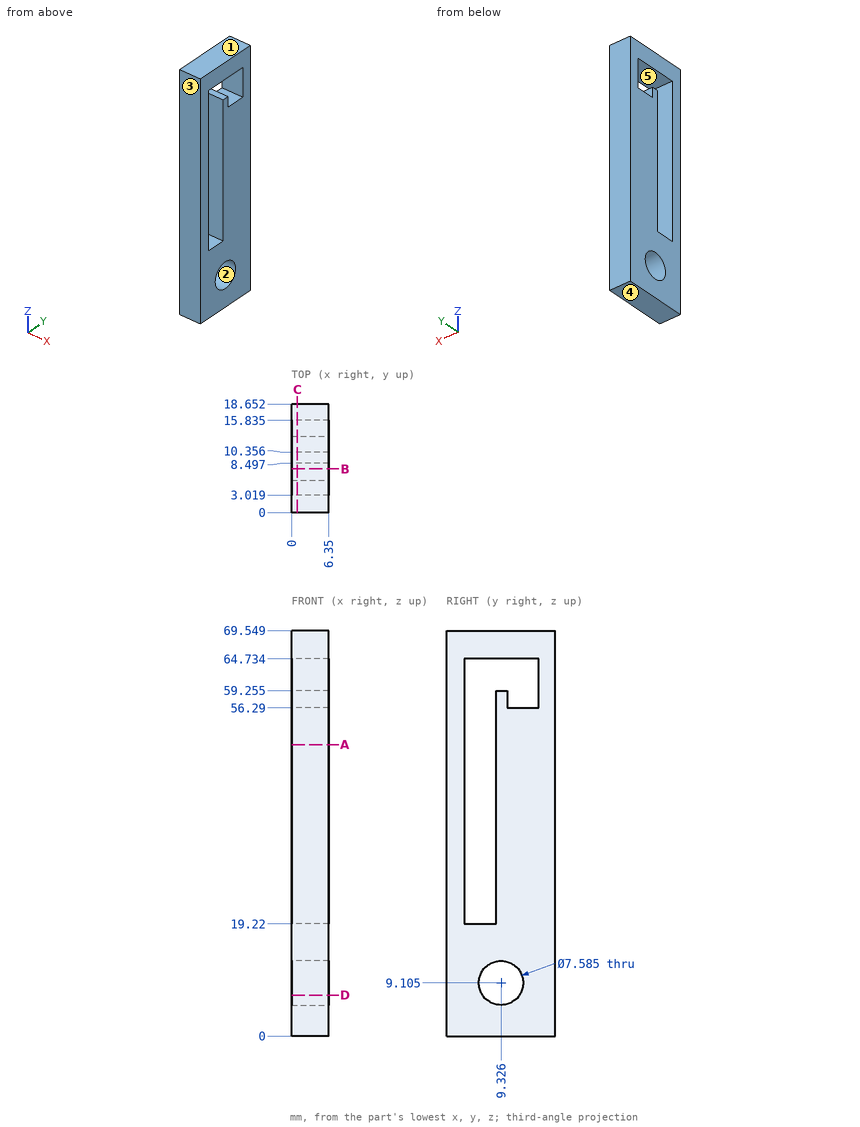
Part print with two shaded views. Sizes in mm from the minimum x, y, z corner. A direction names the side the tool comes from. Round coordinates to 2 decimals unless told otherwise and drop trailing zeros. Write each loop counter-clockwise with the first axis right and the second up, starting at its lowest first coordinate (ties: lowest second). Pieces come first, ordered by that corner, then holes. Notation, with made-up numbers: M -21.5,15 L 37.5,15 A11 cw 37.5,31 Z; hole C -22.75,-10 d7. An arc over 180 degrees is marked long. Put each result on its own line as item: value. Start each with the question number.
1) Pull direction Y, two halves, no side cores. Call the marked faces 1, 2 and 3: pulls with the +Y half, pulls with the -Y half, needs draft (parallel to the pull), parting line crosses it, or undercut.
2) Saw through at D-D, the plane z = 7. Write the cut outline in (x, y).
3) Saw through at A-A, the plane z = 50. Write the cut outline in (x, y).
4) Saw through at B-B, the plane y = 7.5. Write the cut outline in (x, z).
5) Saw through at C-C, the plane x = 1. Count the separate pieces of the cut face and the enclosed holes in it.
6) 3-axis set-ups, long thin cutter, end or side, ignore diameter. For the marked faces 4 and 5: which of +Z, -Z, +X, -X, +Y, -Y reach the whole face in a straight line?
7) Drill centre lines: probe 1 along Y at (x, z) = (2.5, 58) (1 decimal); probe 2 along Y at (x, z) = (5.5, 60.5) (1 decimal); probe 3 along Y at (x, z) = (5.5, 49). Where is each one in solid material? Low to high. Write a range as [from, to].
Resolved:
1. face 1: needs draft
1. face 2: undercut
1. face 3: pulls with the -Y half
2. outline: M 0,0 L 6.35,0 L 6.35,6.17 L 0,6.17 Z; M 0,12.48 L 6.35,12.48 L 6.35,18.65 L 0,18.65 Z
3. outline: M 0,0 L 6.35,0 L 6.35,3.02 L 0,3.02 Z; M 0,8.5 L 6.35,8.5 L 6.35,18.65 L 0,18.65 Z
4. outline: M 0,0 L 6.35,0 L 6.35,5.78 L 0,5.78 Z; M 0,12.43 L 6.35,12.43 L 6.35,19.22 L 0,19.22 Z; M 0,64.73 L 6.35,64.73 L 6.35,69.55 L 0,69.55 Z
5. separate pieces: 1
5. enclosed holes: 2
6. face 4: -Z, +X, -X, +Y, -Y
6. face 5: +X, -X
7. probe 1: [0, 3], [8.5, 10.4], [15.8, 18.7]
7. probe 2: [0, 3], [15.8, 18.7]
7. probe 3: [0, 3.02], [8.5, 18.65]
